Read the model definition and answer for the solid it produces. Units are mm, in the model's axes. A direction names the side the tool comes from. Round coordinates to 2 decimals unless told otherwise and drop trailing zeros. Order: outer loops, then holes, each group sorted by start corner. A loop starts at its lowest first (then second) coordinate and runs counter-clockwise, first axis right, second up.
from build123d import *

# Parameters (mm, degrees)
SKETCH_1_W                  = 10
SKETCH_1_H                  = 20
SKETCH_1_W_2                = 7
SKETCH_1_H_2                = 17
EXTRUDE_1_DEPTH             = 190
HOLE_WIZARD_M31_D           = 2.5
HOLE_WIZARD_M31_DEPTH       = 8.5
HOLE_WIZARD_M31_CSINK_D     = 3.05
HOLE_WIZARD_M31_CSINK_ANGLE = 120
HOLE_WIZARD_M31_TIP         = 0.751075774
HOLE_WIZARD_2_D             = 10
HOLE_WIZARD_2_DEPTH         = 3


with BuildPart() as part:
    # Эскиз1 → Вытянуть-Тонкостенный1 (new body)
    with BuildSketch(Plane.XY):
        with Locations((5, 10)):
            Rectangle(SKETCH_1_W, SKETCH_1_H)
        with Locations((5, 10)):
            Rectangle(SKETCH_1_W_2, SKETCH_1_H_2, mode=Mode.SUBTRACT)
    extrude(amount=EXTRUDE_1_DEPTH)

    # Отверстие обработанное метчиком M31
    with Locations(Plane(origin=(0, 20, 0), x_dir=(-1, 0, 0), z_dir=(0, 1, 0))):
        with Locations((-5, 20), (-5, 57.5), (-5, 95), (-5, 132.5), (-5, 170)):
            CounterSinkHole(HOLE_WIZARD_M31_D / 2, HOLE_WIZARD_M31_CSINK_D / 2, depth=HOLE_WIZARD_M31_DEPTH, counter_sink_angle=HOLE_WIZARD_M31_CSINK_ANGLE)
            with Locations((0, 0, -(HOLE_WIZARD_M31_DEPTH + HOLE_WIZARD_M31_TIP / 2))):  # 118° drill point
                Cone(0, HOLE_WIZARD_M31_D / 2, HOLE_WIZARD_M31_TIP, mode=Mode.SUBTRACT)

    # Отверстие2
    with Locations(Plane(origin=(10, 0, 0), x_dir=(0, 0, -1), z_dir=(1, 0, 0))):
        with Locations((-170, 8), (-120, 8), (-70, 8), (-20, 8)):
            Hole(HOLE_WIZARD_2_D / 2, depth=HOLE_WIZARD_2_DEPTH)


solid = part.part
Q1. Straight lines are drawn through the part: probe 1 along Z at (x, y) = (5, 19.5); probe 2 along Y at (x, z) = (4, 10); probe 3 along X at (y, z) = (11.25, 109). For each, find the intervals that lie inside material, in ascending order.
Outcome:
probe 1: z = 0 to 18.75, 21.25 to 56.25, 58.75 to 93.75, 96.25 to 131.25, 133.75 to 168.75, 171.25 to 190
probe 2: y = 0 to 1.5, 18.5 to 20
probe 3: x = 0 to 1.5, 8.5 to 10
Q2. For a pull along X with two mould halves and no side action, classify faces 4 (the face through (8.5, 10, 94)), 5 (the face through (6.04, 20, 93.67)), 6 (the face through (4, 18.5, 94)), 7 (the face through (10, 10, 94)) as released by +X, released by -X, zero draft, split by the parting line, or undercut.
Outcome:
face 4: undercut
face 5: zero draft
face 6: undercut
face 7: released by +X
Q3. A cutting plane is placed at C-C, the plane z = 70. Give the vertices of the cut face in (x, y), plus the area to 3 significant figures.
Outcome:
outline: (0, 0) - (10, 0) - (10, 3) - (8.5, 3) - (8.5, 1.5) - (1.5, 1.5) - (1.5, 18.5) - (8.5, 18.5) - (8.5, 13) - (10, 13) - (10, 20) - (0, 20) - close
area: 66.0 mm2
Q4. A cutting plane is placed at B-B, the plane y = 16. Give the vertices of the cut face in (x, z).
Outcome:
outline: (0, 0) - (1.5, 0) - (1.5, 190) - (0, 190) - close; (8.5, 0) - (10, 0) - (10, 190) - (8.5, 190) - close
Q5. For faces 1 (the face through (5, 1.5, 94)), 2 (the face through (9.24, 6.085, 124.619)), 3 (the face through (5, 0, 94)), determine the directions among +Z, -Z, +X, -X, +Y, -Y from which every point of the face is accessible in a straight line to the end or side of a thin tool.
Outcome:
face 1: +Z, -Z
face 2: +X
face 3: +Z, -Z, +X, -X, -Y
Q6. Flat-ended cylindrical pins translate along their axes: pin 1 (6 mm diameter, centred on y = 8, z = 20, fed in from +X); pin 2 (2 mm diameter, centred on x = 5, z = 170, fed in from +Y). Find the tip coordinate at first contact, or state that the pin passes through.
Outcome:
pin 1: stops at x = 1.5
pin 2: stops at y = 1.5
Q7. A cutting plane is placed at A-A, the plane z = 39.5. Give the vertices of the cut face in (x, y), plus the area to 3 significant figures.
Outcome:
outline: (0, 0) - (10, 0) - (10, 20) - (0, 20) - close; hole (1.5, 1.5) - (8.5, 1.5) - (8.5, 18.5) - (1.5, 18.5) - close
area: 81.0 mm2
